```python
from build123d import *

# Parameters (mm, degrees)
SKETCH2_R           = 1.5
SKETCH2_R_2         = 3.5
SKETCH2_W           = 71
SKETCH2_H           = 52
BOSS_EXTRUDE1_DEPTH = 2


with BuildPart() as part:
    # Sketch2 → Boss-Extrude1 (new body)
    with BuildSketch(Plane(origin=(0, 0, 0), x_dir=(1, 0, 0), z_dir=(0, 1, 0))):
        with BuildLine():
            Line((-62.225750218, 38.541254469), (67.774249782, 38.541254469))
            ThreePointArc((67.774249782, 38.541254469), (71.309783688, 37.076788375), (72.774249782, 33.541254469))
            Line((72.774249782, 33.541254469), (72.774249782, -36.458745531))
            ThreePointArc((72.774249782, -36.458745531), (71.309783688, -39.994279437), (67.774249782, -41.458745531))
            Line((67.774249782, -41.458745531), (-62.225750218, -41.458745531))
            ThreePointArc((-62.225750218, -41.458745531), (-65.761284124, -39.994279437), (-67.225750218, -36.458745531))
            Line((-67.225750218, -36.458745531), (-67.225750218, 33.541254469))
            ThreePointArc((-67.225750218, 33.541254469), (-65.761284124, 37.076788375), (-62.225750218, 38.541254469))
        make_face()
        with Locations(Location((-58.075750218, 29.791254469, 0), (0, 0, 270))):
            Circle(SKETCH2_R, mode=Mode.SUBTRACT)
        with Locations(Location((63.624249782, 29.791254469, 0), (0, 0, 270))):
            Circle(SKETCH2_R, mode=Mode.SUBTRACT)
        with Locations(Location((-58.075750218, -32.708745531, 0), (0, 0, 270))):
            Circle(SKETCH2_R, mode=Mode.SUBTRACT)
        with Locations(Location((63.624249782, -32.708745531, 0), (0, 0, 270))):
            Circle(SKETCH2_R, mode=Mode.SUBTRACT)
        with Locations(Location((44.830013856, 8.6487321, 0), (0, 0, 270))):
            Circle(SKETCH2_R_2, mode=Mode.SUBTRACT)
        with Locations((-15.575750218, -6.208745531)):
            Rectangle(SKETCH2_W, SKETCH2_H, mode=Mode.SUBTRACT)
    extrude(amount=BOSS_EXTRUDE1_DEPTH)


solid = part.part
```
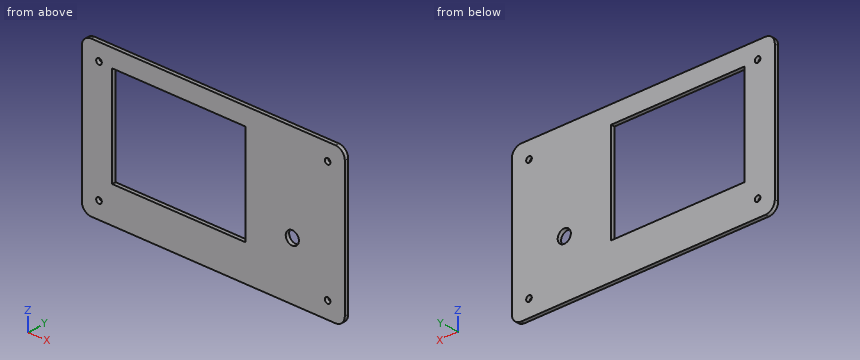
The listing builds one solid part. Answer for the finished solid, in the listing's coordinates (mm). Coordinates: 2 decimals unless noted, no trailing zeros. Loops run counter-clockwise (first coordinate to the right, second up) from the corner with the lowest first, then second, coordinate; pieces in that order, holes last. Notation, with made-up numbers: M 48.5,25.5 L 74.5,25.5 A25 ccw 74.5,43.5 Z; hole C 26,-19.5 d3. An arc over 180 degrees is marked long. Answer as a JSON object with one key per item and string values. Group by question number.
Item 1: Section D-D (y = 0.6) is taken. Write down the section's boundary in (x, z), and give its area (3 significant figures).
Item 2: Section C-C (z = -8) is taken. Write down the section's boundary in (x, y), and give its area (3 significant figures).
Item 3: Section A-A (x = -19.5) is taken. Write down the section's boundary in (y, z), and give its area (3 significant figures).
Item 4: Consider L1, parallel to Z at x = -42, y = 1.6; L2, parallel to X at y = 0.5, z = -2; L3, parallel to Z at x = 44.5, y = 1.65. Determine where each line is inside the solid, lowest interval first.
Item 5: This flat-tipped pin is pushed along its axis until it touches: P1, Ø2.5, axis at x = -58.08, z = 32.71, coming from the +Y side. Where does it stop, or does it pass through?
Item 6: Section B-B (z = 26) is taken. Write down the section's boundary in (x, y).
Solved:
{
 "1": {"outline": "M -67.23,-33.54 A5 ccw -62.23,-38.54 L 67.77,-38.54 A5 ccw 72.77,-33.54 L 72.77,36.46 A5 ccw 67.77,41.46 L -62.23,41.46 A5 ccw -67.23,36.46 Z; hole C -58.08,-29.79 d3; hole C -58.08,32.71 d3; hole M -51.08,-19.79 L 19.92,-19.79 L 19.92,32.21 L -51.08,32.21 Z; hole C 44.83,-8.65 d7; hole C 63.62,-29.79 d3; hole C 63.62,32.71 d3", "area": "7,420 mm2"},
 "2": {"outline": "M -67.23,0 L -51.08,0 L -51.08,2 L -67.23,2 Z; M 19.92,0 L 41.39,0 L 41.39,2 L 19.92,2 Z; M 48.27,0 L 72.77,0 L 72.77,2 L 48.27,2 Z", "area": "124 mm2"},
 "3": {"outline": "M 0,-38.54 L 2,-38.54 L 2,-19.79 L 0,-19.79 Z; M 0,32.21 L 2,32.21 L 2,41.46 L 0,41.46 Z", "area": "56.0 mm2"},
 "4": {"L1": "z = -38.54 to -19.79, 32.21 to 41.46", "L2": "x = -67.23 to -51.08, 19.92 to 72.77", "L3": "z = -38.54 to -12.13, -5.16 to 41.46"},
 "5": {"P1": "passes through"},
 "6": {"outline": "M -67.23,0 L -51.08,0 L -51.08,2 L -67.23,2 Z; M 19.92,0 L 72.77,0 L 72.77,2 L 19.92,2 Z"}
}
